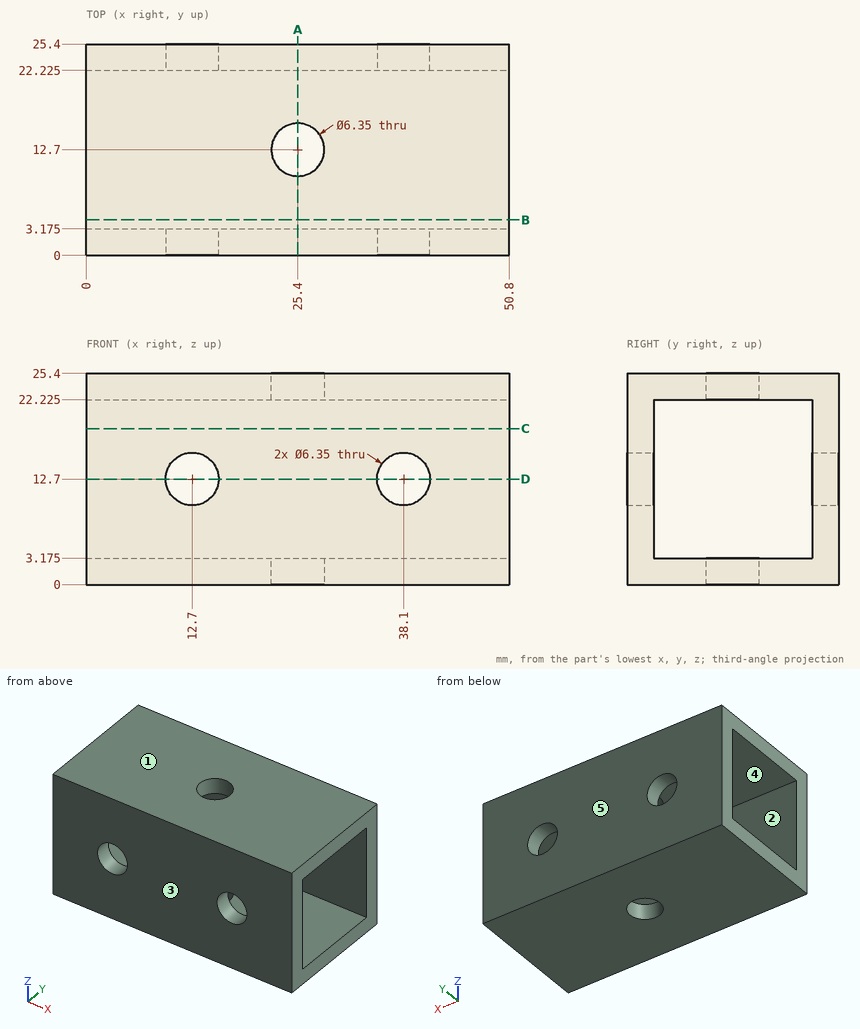
For this review, use the dimensioned drawing (mm, ordinates from the lowest corner) and the shaded views. A direction names the side the tool comes from. Give positions to 0.01 mm unless a question says otherwise; leave off trailing zeros. Order: outer loops, then holes, each group sorted by start corner. A loop starts at its lowest first (then second) coordinate and runs counter-clockwise, first axis right, second up. Notation, with made-up numbers: (58.5, -13) - (109.5, -13) arc R34 cw to (109.5, 18) - close; hole circle Ø6 at (25.5, -40). An arc over 180 degrees is marked (long way). Use a Markdown table: item, result. Add a question column.
(1) Machinability: for the marked faces 4 and 5, which of the approach directions +Z, -Z, +X, -X, +Y, -Y give a long, thin tool a straight path to every point of the face, cutting with its end or side? Answer none if there is none.
(2) Add section D-D on z = 12.7. Give the boundary of the cut face in (x, y) (3 decimals), then the cut area to 3 significant figures.
(3) Add section B-B on y = 4.25. Give the boundary of the cut face in (x, z) (3 decimals).
(4) Add section A-A on x = 25.4. Give the boundary of the cut face in (y, z) (3 decimals).
(5) Mouldability with a two-part tool opening along Y and no side actions: class the marked faces 1, 2 and 3 as +Y half, -Y half, draft (parallel to the pull), parting line (faces both ways), or undercut.
(6) Wall thickness on probe 1 along Y at (x, z) = (32, 14.25) (3 decimals); probe 2 along Z at (x, y) = (38.1, 1.8) (3 decimals): over which ranges is each line inside the solid? List them lowest first. Write a range as [from, to].
Report:
| question | item | result |
|---|---|---|
| 1 | face 4 | +X, -X |
| 1 | face 5 | +Z, -Z, +X, -X, +Y |
| 2 | outline | (0, 0) - (9.525, 0) - (9.525, 3.175) - (0, 3.175) - close; (0, 22.225) - (9.525, 22.225) - (9.525, 25.4) - (0, 25.4) - close; (15.875, 0) - (34.925, 0) - (34.925, 3.175) - (15.875, 3.175) - close; (15.875, 22.225) - (34.925, 22.225) - (34.925, 25.4) - (15.875, 25.4) - close; (41.275, 0) - (50.8, 0) - (50.8, 3.175) - (41.275, 3.175) - close; (41.275, 22.225) - (50.8, 22.225) - (50.8, 25.4) - (41.275, 25.4) - close |
| 2 | area | 242 mm² |
| 3 | outline | (0, 0) - (50.8, 0) - (50.8, 3.175) - (0, 3.175) - close; (0, 22.225) - (50.8, 22.225) - (50.8, 25.4) - (0, 25.4) - close |
| 4 | outline | (0, 0) - (9.525, 0) - (9.525, 3.175) - (3.175, 3.175) - (3.175, 22.225) - (9.525, 22.225) - (9.525, 25.4) - (0, 25.4) - close; (15.875, 0) - (25.4, 0) - (25.4, 25.4) - (15.875, 25.4) - (15.875, 22.225) - (22.225, 22.225) - (22.225, 3.175) - (15.875, 3.175) - close |
| 5 | face 1 | draft |
| 5 | face 2 | undercut |
| 5 | face 3 | -Y half |
| 6 | probe 1 | y = [0, 3.175], [22.225, 25.4] |
| 6 | probe 2 | z = [0, 9.525], [15.875, 25.4] |
